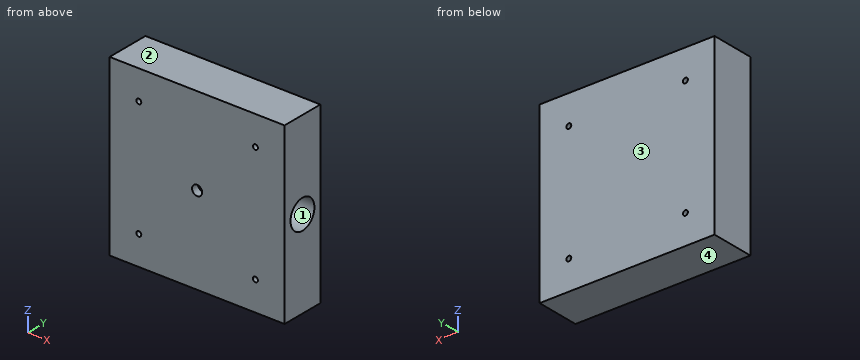
```python
from build123d import *

# Parameters (mm, degrees)
F0_W     = 152.4
F0_H     = 152.4
F1_DEPTH = 38.1
F4_D     = 8.7376
F4_DEPTH = 12.7
F4_TIP   = 2.6250398724
F2_R     = 12.7
F5_DEPTH = 127
F7_D     = 4.318
F7_DEPTH = 38.1
F7_TIP   = 1.2972580765


with BuildPart() as f1:
    # F0 (on Front) → F1 (new body)
    with BuildSketch(Plane.XZ):
        Rectangle(F0_W, F0_H)
    extrude(amount=F1_DEPTH)

    # F4
    with Locations(Plane.XZ.offset(38.1)):
        with Locations((0, 0)):
            Hole(F4_D / 2, depth=F4_DEPTH)
            with Locations((0, 0, -(F4_DEPTH + F4_TIP / 2))):  # 118° drill point
                Cone(0, F4_D / 2, F4_TIP, mode=Mode.SUBTRACT)

    # F2 (on face) → F5 (cut)
    with BuildSketch(Plane.YZ.offset(76.2)):
        with Locations((-19.05, 0)):
            Circle(F2_R)
    extrude(amount=-F5_DEPTH, mode=Mode.SUBTRACT)

    # F7
    with Locations(Plane.XZ.offset(38.1)):
        with Locations((-50.8, 50.8), (50.8, 50.8), (-50.8, -50.8), (50.8, -50.8)):
            Hole(F7_D / 2, depth=F7_DEPTH)
            with Locations((0, 0, -(F7_DEPTH + F7_TIP / 2))):  # 118° drill point
                Cone(0, F7_D / 2, F7_TIP, mode=Mode.SUBTRACT)


solid = f1.part
```
Read the model definition and answer for the solid it produces. Units are mm, in the model's axes. Face numbers are marked on the shaded views. Give positions to 0.01 mm unless a question says otherwise; leave off trailing zeros. Order: outer loops, then holes, each group sorted by start corner. A loop starts at its lowest first (then second) coordinate and runs counter-clockwise, first axis right, second up.
(1) For a pull along Z with two mould halves and no side action, classify the marked faces 1, 2, 3 and 4 as released by +Z, released by -Z, zero draft, split by the parting line, or undercut.
(2) Straight lines are drawn through the part: L1, parallel to X at y = -19.5, z = -50.8; L2, parallel to Z at x = 0, y = -33; L3, parallel to Z at x = 50, y = -16. For each, find the intervals that lie inside material, in ascending order.
(3) Find section D-D (y = -19.05). Give the vertices of the cut face in (x, z).
(4) Given pin 1 (11.5 mm diameter, centred on x = 0, z = 0, fed in from -Y), flat-ended and moving along its own axis, determine where the tip first touches the part or whether it passes through.
(5) Find section B-B (z = 50.8). Give the vertices of the cut face in (x, y).
(6) Find section C-C (z = 0). Give the vertices of the cut face in (x, y), plus the area to 3 significant figures.
(7) Find section A-A (x = 50.8). Give the vertices of the cut face in (y, z).
Result sheet:
1. face 1: undercut
1. face 2: released by +Z
1. face 3: zero draft
1. face 4: released by -Z
2. L1: x = -76.2 to -52.96, -48.64 to 48.64, 52.96 to 76.2
2. L2: z = -76.2 to -4.37, 4.37 to 76.2
2. L3: z = -76.2 to -52.81, -48.79 to -12.33, 12.33 to 48.79, 52.81 to 76.2
3. outline: (-76.2, -76.2) - (76.2, -76.2) - (76.2, -12.7) - (-50.8, -12.7) - (-50.8, 12.7) - (76.2, 12.7) - (76.2, 76.2) - (-76.2, 76.2) - close; hole circle Ø4.32 at (-50.8, -50.8); hole circle Ø4.32 at (-50.8, 50.8); hole circle Ø4.32 at (50.8, -50.8); hole circle Ø4.32 at (50.8, 50.8)
4. pin 1: stops at y = -38.1
5. outline: (-76.2, -38.1) - (-52.96, -38.1) - (-52.96, 0) - (-76.2, 0) - close; (-48.64, -38.1) - (48.64, -38.1) - (48.64, 0) - (-48.64, 0) - close; (52.96, -38.1) - (76.2, -38.1) - (76.2, 0) - (52.96, 0) - close
6. outline: (-76.2, -38.1) - (-4.37, -38.1) - (-4.37, -31.75) - (-50.8, -31.75) - (-50.8, -6.35) - (76.2, -6.35) - (76.2, 0) - (-76.2, 0) - close; (4.37, -38.1) - (76.2, -38.1) - (76.2, -31.75) - (4.37, -31.75) - close
6. area: 2,530 mm2
7. outline: (-38.1, -76.2) - (0, -76.2) - (0, -52.96) - (-38.1, -52.96) - close; (-38.1, -48.64) - (0, -48.64) - (0, 48.64) - (-38.1, 48.64) - close; (-38.1, 52.96) - (0, 52.96) - (0, 76.2) - (-38.1, 76.2) - close; hole circle Ø25.4 at (-19.05, 0)
